Autodesk Inventor part; units mm, degrees
ref_plane "YZ Plane" through (0, 0, 0) normal (1, 0, 0) x (0, 1, 0)
ref_plane "XZ Plane" through (0, 0, 0) normal (0, 1, 0) x (-1, 0, 0)
ref_plane "XY Plane" through (0, 0, 0) normal (0, 0, 1) x (1, 0, 0)
sketch "Sketch1" plane through (0, 0, 0) normal (1, 0, 0) x (0, 1, 0)
  line L0 (-9.1, 5) -> (9.1, 5)
  line L1 (9.1, 5) -> (9.1, -5)
  line L2 (9.1, -5) -> (-9.1, -5)
  line L3 (-9.1, -5) -> (-9.1, 5)
  line L4 (-9.1, 5) -> (9.1, -5) construction
  line L5 (9.1, 5) -> (-9.1, -5) construction
  point P0 (0, 0)
  dimension "d0" = 18.2
  dimension "d1" = 10
extrude "Extrusion1" add sketch "Sketch1" along normal blind 10
sketch "Sketch2" plane through (0, 9.1, 5) normal (0, 1, 0) x (1, 0, 0)
  line L0 (0, 5) -> (5, 5)
  circle A0 centre (5, 5) radius 2
  dimension "d4" = 5
  dimension "d5" = 4
extrude "Extrusion2" cut sketch "Sketch2" against normal blind 8
thread "Thread1"
sketch "Sketch3" plane through (0, -9.1, -5) normal (0, -1, 0) x (1, 0, 0)
  line L0 (0, 5) -> (5, 5)
  circle A0 centre (5, 5) radius 2
  dimension "d10" = 5
  dimension "d11" = 4
extrude "Extrusion3" cut sketch "Sketch3" against normal blind 8
thread "Thread2"
properties part number "Rb PEEK - Soporte"
Design review of the part built by this model. Coordinates are the model's own, in mm. A direction names the side the tool comes from. Give positions to 0.01 mm unless a question says otherwise; leave off trailing zeros. Write each loop counter-clockwise with the first axis right and the second up, starting at its lowest first coordinate (ties: lowest second). Pieces come first, ordered by that corner, then holes.
(1) Wall thickness on line 1 along Z through (x, y) = (5, -2.5); line 2 along X through (y, z) = (-5, 0); line 3 along Y through (x, z) = (6.25, -1.25): over which ranges is each line inside the solid? List them lowest first.
Checked values:
line 1: z = -5 to -2, 2 to 5
line 2: x = 0 to 3, 7 to 10
line 3: y = -1.1 to 1.1
(2) Add section B-B (z = 0). Give the boundary of the cut face in (x, y), and give its area (3 significant figures).
Checked values:
outline: (0, -9.1) - (3, -9.1) - (3, -1.1) - (7, -1.1) - (7, -9.1) - (10, -9.1) - (10, 9.1) - (7, 9.1) - (7, 1.1) - (3, 1.1) - (3, 9.1) - (0, 9.1) - close
area: 118 mm2
(3) Add section A-A (y = 5.25). Give the boundary of the cut face in (x, z).
Checked values:
outline: (0, -5) - (10, -5) - (10, 5) - (0, 5) - close; hole circle Ø4 at (5, 0)
(4) Add section C-C (x = 5.75). Give the boundary of the cut face in (y, z), and give its area (3 significant figures).
Checked values:
outline: (-9.1, -5) - (9.1, -5) - (9.1, -1.85) - (1.1, -1.85) - (1.1, 1.85) - (9.1, 1.85) - (9.1, 5) - (-9.1, 5) - (-9.1, 1.85) - (-1.1, 1.85) - (-1.1, -1.85) - (-9.1, -1.85) - close
area: 123 mm2
(5) Mouldability with a two-part tool opening along X and no side actions: class faces 1 (the face through (5, -1.1, 0)), 2 (the face through (5, 0, 5)), 3 (the face through (0, 0, 0)) as +X half, -X half, draft (parallel to the pull), parting line (faces both ways), or undercut.
Checked values:
face 1: undercut
face 2: draft
face 3: -X half
(6) Tool access review of faces 4 (the face through (5, 1.1, 0)), 5 (the face through (3, -5, 0)), 6 (the face through (2.7, 9.1, 0.1)): name each direction out of +Z, -Z, +X, -X, +Y, -Y from which nothing blocks a thin tool from reaching the whole face with its end or side.
Checked values:
face 4: +Y
face 5: -Y
face 6: +Z, -Z, +X, -X, +Y
(7) Clearance check with a flat-ended pin moving along its axis: pin 1 Ø3 at (x, z) = (5, 0) entering from +Y. State where the tip first meets the part, or that it passes through.
Checked values:
pin 1: stops at y = 1.1
